Model file for the job. Use its own axes, mm. A direction names the side the tool comes from. Round coordinates to 2 decimals unless told otherwise and drop trailing zeros. Loops run counter-clockwise (first coordinate to the right, second up) from the corner with the lowest first, then second, coordinate; pieces in that order, holes last. Notation, with made-up numbers: M 40.25,69 L 97.25,69 A22 cw 97.25,80 Z; hole C 4.5,60.25 d3. An arc over 180 degrees is marked long. Use a Markdown table: item, result. Add a question column.
Item 1: Two-plate mould, pull along X, no slides. Class faces 1 (the flat face through (26.586, 0, -11)), 2 (the cylindrical face through (62.834, -0.007, -10.324)), 3 (the flat face through (18.586, 0, 10)), 4 (the flat face through (15.671, -0.007, -18.514)): +X half, -X half, draft (parallel to the pull), parting line (faces both ways), or undercut.
Item 2: Saw through at B-B on z = 6. Write the cut outline in (x, y).
Item 3: Tool access for faces 5 (the flat face through (55.56, -0.01, 14.65)), 6 (the flat face through (23, 0, 13)), 7 (the flat face through (63, 0, 2.275)): list every direction of +Z, -Z, +X, -X, +Y, -Y with a clear straight run to the whole face (end or side of a thin tool).
Item 4: Saw through at A-A on x = 48.5. Write the cut outline in (y, z).
Item 5: Saw through at C-C on z = 0. Write the cut outline in (x, y).
Item 6: Pin check, flat tips, straight feed: P1, Ø0.5, axis at y = 0, z = -9.5, coming from the +X side; P2, Ø0.5, axis at x = 15, y = 0, coming from the -Z side; P3, Ø0.5, axis at y = 0, z = 1.5, coming from the -X side; P4, Ø2, axis at x = 20.5, z = -8.5, coming from the -Y side. Stop position of each tip, or through.
Item 7: Wall check: L1, parallel to Z at x = 20.5, y = 0.05; L2, parallel to Z at x = 26.5, y = -0.25; L3, parallel to X at y = -0.2, z = 9.5. Give the ranges that are in metal, low to high. Write a range as from..to.
```python
from build123d import *

# Parameters (mm, degrees)
F1_DEPTH = 0.5


# Not quite as in the source:
# - ends of sketch curves that miss each other by under 0.0002 mm in the source are joined


with BuildPart() as f1:
    # F0 (on Front) → F1 (new body, symmetric)
    with BuildSketch(Plane.XZ):
        with BuildLine():
            Line((53.992555, -15.220268), (57.083133, -14.095389))
            ThreePointArc((57.083133, -14.095389), (62.9018568836, -10.252747544), (66.3544503107, -4.1944440905))
            ThreePointArc((66.3544503107, -4.1944440905), (66.1141142416, -2.8747683688), (64.914288, -2.275))
            Line((64.914288, -2.275), (60.670593, -2.275))
            ThreePointArc((60.670593, -2.275), (59.8472095147, -2.5211899521), (59.2941043505, -3.1789471518))
            ThreePointArc((59.2941043505, -3.1789471518), (56.9827494729, -6.2209259886), (53.52425904, -7.8441451998))
            ThreePointArc((53.52425904, -7.8441451998), (52.6431740995, -8.0626756758), (51.7855370008, -8.3602070021))
            ThreePointArc((51.7855370008, -8.3602070021), (39.452831, 0), (51.7855371982, 8.3602074972))
            ThreePointArc((51.7855371982, 8.3602074972), (52.6431743712, 8.0626765952), (53.524259133, 7.844145664))
            ThreePointArc((53.524259133, 7.844145664), (56.9827494729, 6.2209259886), (59.2941043849, 3.1789471667))
            ThreePointArc((59.2941043849, 3.1789471667), (59.8472095147, 2.5211899521), (60.670593, 2.275))
            Line((60.670593, 2.275), (64.914288, 2.275))
            ThreePointArc((64.914288, 2.275), (66.1141145297, 2.8747687527), (66.3544497778, 4.1944449353))
            ThreePointArc((66.3544497778, 4.1944449353), (62.9018565554, 10.2527478944), (57.0831331177, 14.0953893235))
            Line((57.0831331177, 14.0953893235), (53.992555, 15.220268))
            ThreePointArc((53.992555, 15.220268), (52.3736165632, 15.715360306), (50.7118440801, 16.0387645685))
            Line((50.7118440801, 16.0387645685), (40.585713, 17.465))
            Line((40.585713, 17.465), (35.885713, 17.465))
            ThreePointArc((35.885713, 17.465), (35.6735809656, 17.5528679656), (35.585713, 17.765))
            Line((35.585713, 17.765), (35.585713, 18.7))
            ThreePointArc((35.585713, 18.7), (35.4978450344, 18.9121320344), (35.285713, 19))
            Line((35.285713, 19), (18.585713, 19))
            Line((18.585713, 19), (12.836393, 18.04178))
            ThreePointArc((12.836393, 18.04178), (12.656806899, 17.9397743434), (12.585713, 17.745862))
            Line((12.585713, 17.745862), (12.585713, 6.875))
            ThreePointArc((12.585713, 6.875), (12.6735809656, 6.6628679656), (12.885713, 6.575))
            Line((12.885713, 6.575), (18.285713, 6.575))
            ThreePointArc((18.285713, 6.575), (18.4978450344, 6.6628679656), (18.585713, 6.875))
            Line((18.585713, 6.875), (18.585713, 12.7))
            ThreePointArc((18.585713, 12.7), (18.6735809656, 12.9121320344), (18.885713, 13))
            Line((18.885713, 13), (26.285713, 13))
            ThreePointArc((26.285713, 13), (26.4978450344, 12.9121320344), (26.585713, 12.7))
            Line((26.585713, 12.7), (26.585713, 10.3))
            ThreePointArc((26.585713, 10.3), (26.6735809656, 10.0878679656), (26.885713, 10))
            Line((26.885713, 10), (32.285713, 10))
            ThreePointArc((32.285713, 10), (32.4978450344, 9.9121320344), (32.585713, 9.7))
            Line((32.585713, 9.7), (32.585713, -9.7))
            ThreePointArc((32.585713, -9.7), (32.4978450344, -9.9121320344), (32.285713, -10))
            Line((32.285713, -10), (26.885713, -10))
            ThreePointArc((26.885713, -10), (26.6735809656, -10.0878679656), (26.585713, -10.3))
            Line((26.585713, -10.3), (26.585713, -12.7))
            ThreePointArc((26.585713, -12.7), (26.4978450344, -12.9121320344), (26.285713, -13))
            Line((26.285713, -13), (18.885713, -13))
            ThreePointArc((18.885713, -13), (18.6735809656, -12.9121320344), (18.585713, -12.7))
            Line((18.585713, -12.7), (18.585713, -6.875))
            ThreePointArc((18.585713, -6.875), (18.4978450344, -6.6628679656), (18.285713, -6.575))
            Line((18.285713, -6.575), (12.885713, -6.575))
            ThreePointArc((12.885713, -6.575), (12.6735809656, -6.6628679656), (12.585713, -6.875))
            Line((12.585713, -6.875), (12.585713, -17.745862))
            ThreePointArc((12.585713, -17.745862), (12.656806899, -17.9397743434), (12.8363929795, -18.0417801231))
            Line((12.8363929795, -18.0417801231), (18.585713, -19))
            Line((18.585713, -19), (35.285713, -19))
            ThreePointArc((35.285713, -19), (35.4978450344, -18.9121320344), (35.585713, -18.7))
            Line((35.585713, -18.7), (35.585713, -17.765))
            ThreePointArc((35.585713, -17.765), (35.6735809656, -17.5528679656), (35.885713, -17.465))
            Line((35.885713, -17.465), (40.585713, -17.465))
            Line((40.585713, -17.465), (50.711844, -16.038764))
            ThreePointArc((50.711844, -16.038764), (52.3736165632, -15.715360306), (53.992555, -15.220268))
        make_face()
    extrude(amount=F1_DEPTH, both=True)


solid = f1.part
```
Entries:
| question | item | result |
|---|---|---|
| 1 | face 1 | undercut |
| 1 | face 2 | +X half |
| 1 | face 3 | undercut |
| 1 | face 4 | -X half |
| 2 | outline | M 32.59,-0.5 L 41.74,-0.5 L 41.74,0.5 L 32.59,0.5 Z; M 57.24,-0.5 L 65.7,-0.5 L 65.7,0.5 L 57.24,0.5 Z |
| 3 | face 5 | +Z, +X, +Y, -Y |
| 3 | face 6 | +Y, -Y |
| 3 | face 7 | +X, +Y, -Y |
| 4 | outline | M -0.5,-16.35 L 0.5,-16.35 L 0.5,-9 L -0.5,-9 Z; M -0.5,9 L 0.5,9 L 0.5,16.35 L -0.5,16.35 Z |
| 5 | outline | M 32.59,-0.5 L 39.45,-0.5 L 39.45,0.5 L 32.59,0.5 Z |
| 6 | P1 | x = 63.76 |
| 6 | P2 | z = -18.44 |
| 6 | P3 | x = 32.59 |
| 6 | P4 | through |
| 7 | L1 | -19..-13, 13..19 |
| 7 | L2 | -19..-12.91, 12.91..19 |
| 7 | L3 | 12.59..18.59, 32.59..63.56 |
